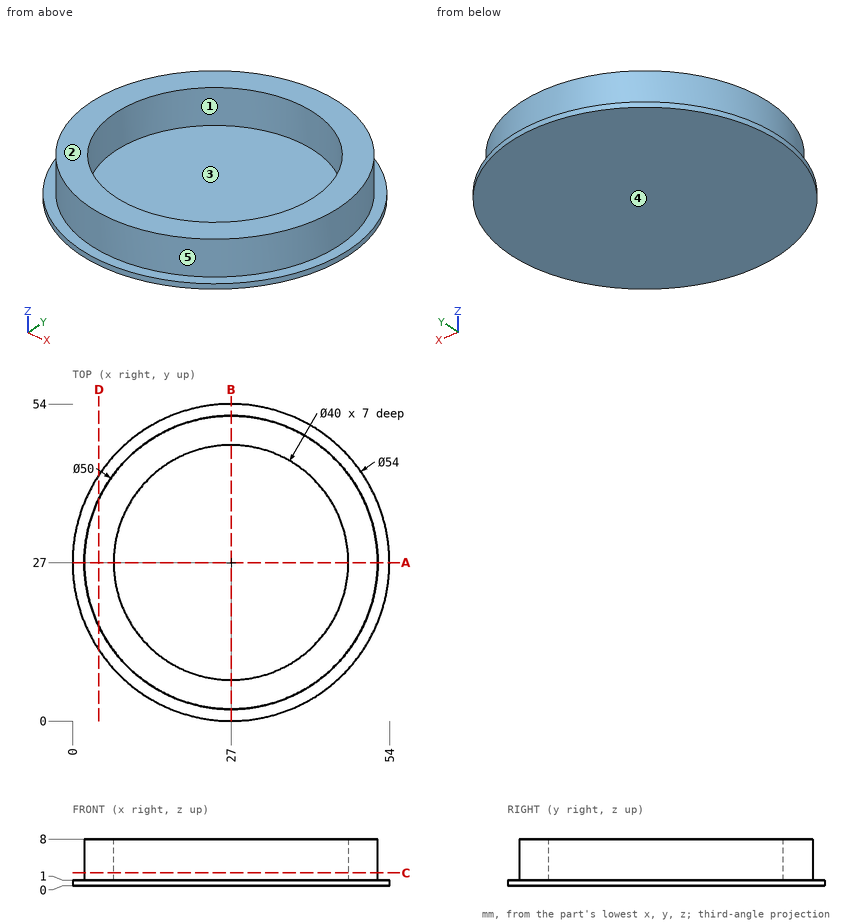
Can you work these out from the drawing? Everything is in mm from the part's minimum corner. A direction names the side the tool comes from. Coordinates: 2 decimals unless noted, no trailing zeros. Loops run counter-clockwise (first coordinate to the right, second up) from the corner with the lowest first, then second, coordinate; pieces in that order, holes last.
1. I need wall thicknesses on L1, parallel to Y at x = 27, z = 5; L2, parallel to Z at x = 17, y = 12; L3, parallel to X at y = 15.5, z = 4.75. Which ranges of each line are inside material? Lowest first, please.
2. Imagine slicing it at D-D, the plane x = 4.5. Please give me the cut outline in (y, z), and give its area (3 significant figures).
3. Imagine slicing it at C-C, the plane z = 2.25. Please give me the cut outline in (x, y).
4. For the marked faces 1 and 2, which set-ups out of +Z, -Z, +X, -X, +Y, -Y let a thin tool reach every point of the face, with its end or its side?
5. Imagine slicing it at A-A, the plane y = 27. Please give me the cut outline in (x, z).
6. For P1, Ø1.5, axis at x = 12.5, z = 5.5, coming from the +Y side; P2, Ø12, axis at x = 13, y = 40, coming from the -Z side; P3, Ø1.5, axis at y = 26, z = 7, coming from the +X side; P4, Ø1.5, axis at y = 34.5, z = 5, coming from the +X side, each with a flat end and sliding along its axis, tell me the tip position at first contact or that it passes through.
7. If we mould it in two halves opening along Y, with no side actions, what happens to the marked faces 3, 4 and 5? For each: pulls with the +Y half, pulls with the -Y half, needs draft (parallel to the pull), parting line crosses it, or undercut.
Taken from the geometry:
1. L1: y = 2 to 7, 47 to 52
1. L2: z = 0 to 1
1. L3: x = 4.8 to 10.64, 43.36 to 49.2
2. outline: (12.08, 0) - (41.92, 0) - (41.92, 1) - (37.9, 1) - (37.9, 8) - (16.1, 8) - (16.1, 1) - (12.08, 1) - close
2. area: 182 mm2
3. outline: circle Ø50 at (27, 27); hole circle Ø40 at (27, 27)
4. face 1: +Z
4. face 2: +Z, +X, -X, +Y, -Y
5. outline: (0, 0) - (54, 0) - (54, 1) - (52, 1) - (52, 8) - (47, 8) - (47, 1) - (7, 1) - (7, 8) - (2, 8) - (2, 1) - (0, 1) - close
6. P1: stops at y = 47.88
6. P2: stops at z = 0
6. P3: stops at x = 52
6. P4: stops at x = 51.07
7. face 3: undercut
7. face 4: needs draft
7. face 5: parting line crosses it
